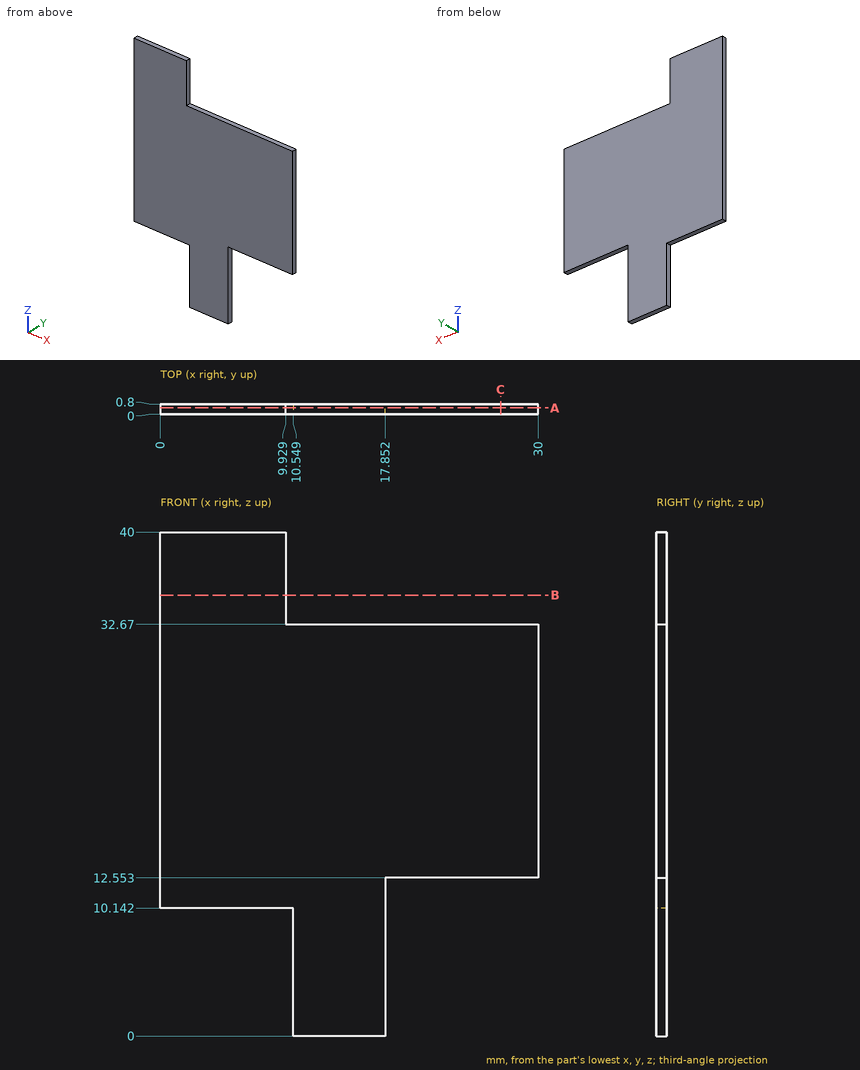
Here's the drawing with two shaded views (mm, measured from the low corner). I have some questions. Give positions to 0.01 mm unless a question says otherwise; leave off trailing zeros. Loops run counter-clockwise (first coordinate to the right, second up) from the corner with the lowest first, then second, coordinate; pieces in that order, holes last. Notation, with made-up numbers: M 61.25,-5.75 L 65.25,-5.75 A29 cw 65.25,29.25 Z; hole C 32.25,1.25 d1. An arc over 180 degrees is marked long. Answer in a Markdown table with one row per item.
1. Suppose I cut it at B-B on z = 35. Write out the boundary of the cut face in (x, y).
Taken from the geometry:
| item | result |
|---|---|
| outline | M 0,0 L 9.93,0 L 9.93,0.8 L 0,0.8 Z |
2. Suppose I cut it at A-A on y = 0.5. Write out the boundary of the cut face in (x, z), plus the area to 3 significant figures.
Taken from the geometry:
| item | result |
|---|---|
| outline | M 0,10.14 L 10.55,10.14 L 10.55,0 L 17.85,0 L 17.85,12.55 L 30,12.55 L 30,32.67 L 9.93,32.67 L 9.93,40 L 0,40 Z |
| area | 793 mm² |
3. Suppose I cut it at C-C on x = 27. Write out the boundary of the cut face in (y, z), plus the area to 3 significant figures.
Taken from the geometry:
| item | result |
|---|---|
| outline | M 0,12.55 L 0.8,12.55 L 0.8,32.67 L 0,32.67 Z |
| area | 16.1 mm² |
4. If I drill on line 1 along Z through (x, y) = (2.75, 0.35); line 2 along Z through (x, y) = (26.25, 0.55); line 3 along X through (y, z) = (0.45, 12.5), over which ranges is the centre line in solid material (lowest first)?
Taken from the geometry:
| item | result |
|---|---|
| line 1 | z = 10.14 to 40 |
| line 2 | z = 12.55 to 32.67 |
| line 3 | x = 0 to 17.85 |
